from build123d import *

# Parameters (mm, degrees)
F0_R     = 37.5
F1_DEPTH = 120
F3_DEPTH = 115
F4_W     = 70
F4_H     = 33
F5_DEPTH = 40
F6_W     = 5
F6_H     = 70
F7_DEPTH = 109


with BuildPart() as f1:
    # F0 (on Top) → F1 (new body)
    with BuildSketch(Plane.XY):
        Circle(F0_R)
    extrude(amount=F1_DEPTH)

    # F2 (on face) → F3 (cut)
    with BuildSketch(Plane.XY.offset(120)):
        with BuildLine():
            Line((0, -35), (0, 35))
            ThreePointArc((0, 35), (-24.748737, 24.748737), (-35, 0))
            ThreePointArc((-35, 0), (-24.748737, -24.748737), (0, -35))
        make_face()
    extrude(amount=-F3_DEPTH, mode=Mode.SUBTRACT)

    # F4 (on face) → F5 (cut)
    with BuildSketch(Plane(origin=(0, 0, 0), x_dir=(0, -1, 0), z_dir=(-1, 0, 0))):
        with Locations((0, 22.5)):
            Rectangle(F4_W, F4_H)
        with Locations((0, 60.5)):
            Rectangle(F4_W, F4_H)
        with Locations((0, 98.5)):
            Rectangle(F4_W, F4_H)
    extrude(amount=-F5_DEPTH, mode=Mode.SUBTRACT)

    # F6 (on face) → F7 (join)
    with BuildSketch(Plane.XY.offset(6)):
        with Locations((2.5, 0)):
            Rectangle(F6_W, F6_H)
    extrude(amount=F7_DEPTH)


solid = f1.part
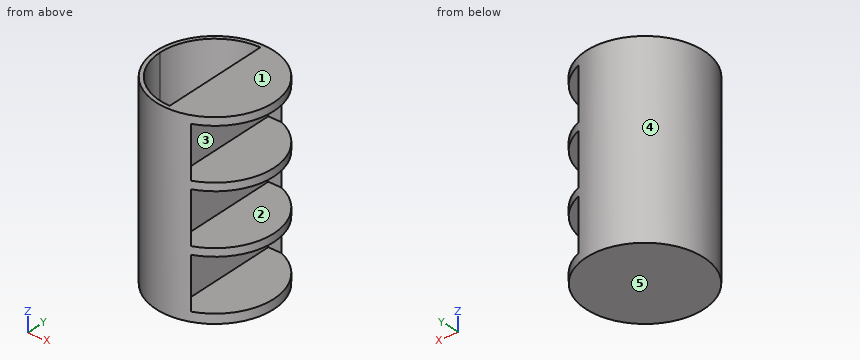
Check sheet for the modelled part. Datum: model origin and axes. Units: mm. Face numbers are marked on the shaded views. A direction names the side the tool comes from. Round coordinates to 2 decimals unless told otherwise and drop trailing zeros. Order: outer loops, then holes, each group sorted by start corner. A loop starts at its lowest first (then second) coordinate and runs counter-clockwise, first axis right, second up.
Q1. Draft check along Y on the marked faces 3, 4 and 5. Enter one of: pulls with the +Y half, pulls with the -Y half, needs draft (parallel to the pull), parting line crosses it, or undercut.
Filled sheet:
face 3: undercut
face 4: parting line crosses it
face 5: needs draft
Q2. Depth check by flat-ended pin: P1, Ø1, axis at x = 11.5, z = 91.5, coming from the +Y side; P2, Ø9.5, axis at x = 10, z = 60, coming from the -Y side; P3, Ø1.5, axis at y = -6.5, z = 82.5, coming from the -X side; P4, Ø5, axis at x = -2, y = 23.5, coming from the -Z side. Enter the tip coordinate at first touch or a pass-through.
Filled sheet:
P1: stops at y = 35.85
P2: stops at y = -37.13
P3: stops at x = -37.06
P4: stops at z = 0
Q3. Set-up check for the marked faces 1 and 2: record each of +Z, -Z, +X, -X, +Y, -Y from which the full face is reachable in a straight line by a thin tool's end or side.
Filled sheet:
face 1: +Z, +X, -X, +Y, -Y
face 2: +X
Q4. Cross-section at B-B, the plane y = 14. Enter the section's corners in (x, z), plus the area to 3 significant figures.
Filled sheet:
outline: (-34.79, 0) - (34.79, 0) - (34.79, 6) - (5, 6) - (5, 39) - (34.79, 39) - (34.79, 44) - (5, 44) - (5, 77) - (34.79, 77) - (34.79, 82) - (5, 82) - (5, 115) - (34.79, 115) - (34.79, 120) - (0, 120) - (0, 5) - (-32.08, 5) - (-32.08, 120) - (-34.79, 120) - close
area: 1,710 mm2
Q5. Cross-section at A-A, the plane z = 68. Enter the section's corners in (x, y).
Filled sheet:
outline: (5, -35) - (5, 35) - (13.46, 35) arc R37.5 ccw (long way) to (13.46, -35) - close; hole (-35, 0) arc R35 ccw to (0, -35) - (0, 35) arc R35 ccw to start
Q6. Scan lines: L1, parallel to Z at x = 25.5, y = -18; L2, parallel to X at y = -1, z = 70.5; L3, parallel to Z at x = -2, y = 1. Record each from-to range of solid material in increasing order.
Filled sheet:
L1: z = 0 to 6, 39 to 44, 77 to 82, 115 to 120
L2: x = -37.49 to -34.99, 0 to 5
L3: z = 0 to 5
Q7. Cross-section at C-C, the plane y = -16. Enter the section's corners in (x, z), plus the area to 3 significant figures.
Filled sheet:
outline: (-33.92, 0) - (33.92, 0) - (33.92, 6) - (5, 6) - (5, 39) - (33.92, 39) - (33.92, 44) - (5, 44) - (5, 77) - (33.92, 77) - (33.92, 82) - (5, 82) - (5, 115) - (33.92, 115) - (33.92, 120) - (0, 120) - (0, 5) - (-31.13, 5) - (-31.13, 120) - (-33.92, 120) - close
area: 1,700 mm2
